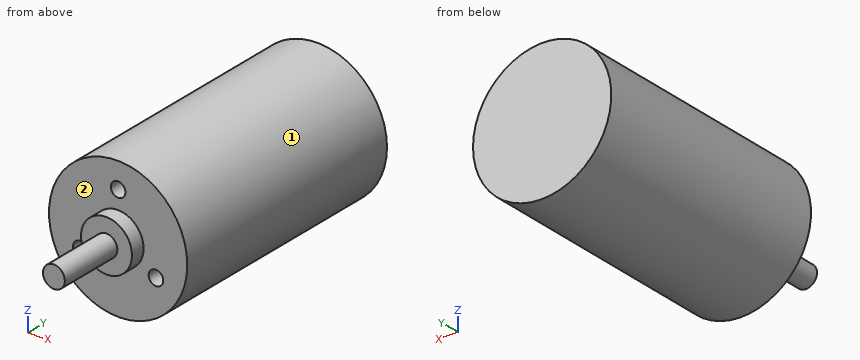
from build123d import *

# Parameters (mm, degrees)
F0_R     = 9.5
F1_DEPTH = 34.2
F2_R     = 3.5
F3_DEPTH = 2
F4_R     = 1.5
F5_DEPTH = 9
F7_D     = 2
F7_DEPTH = 3
F7_TIP   = 0.600860619


with BuildPart() as f1:
    # F0 (on Front) → F1 (new body)
    with BuildSketch(Plane.XZ):
        Circle(F0_R)
    extrude(amount=F1_DEPTH)

    # F2 (on face) → F3 (join)
    with BuildSketch(Plane.XZ.offset(34.2)):
        Circle(F2_R)
    extrude(amount=F3_DEPTH)

    # F4 (on face) → F5 (join)
    with BuildSketch(Plane.XZ.offset(36.2)):
        Circle(F4_R)
    extrude(amount=F5_DEPTH)

    # F7
    with Locations(Plane.XZ.offset(34.2)):
        with Locations((0, 6), (-5.1961524227, -3), (5.1961524227, -3)):
            Hole(F7_D / 2, depth=F7_DEPTH)
            with Locations((0, 0, -(F7_DEPTH + F7_TIP / 2))):  # 118° drill point
                Cone(0, F7_D / 2, F7_TIP, mode=Mode.SUBTRACT)


solid = f1.part
Could you check a few things on this model? Use its own coordinates, in mm. Face numbers are marked on the shaded views. A direction names the side the tool comes from. Coordinates: 2 decimals unless noted, no trailing zeros. Write each loop counter-clockwise with the first axis right and the second up, starting at its lowest first coordinate (ties: lowest second). Pieces come first, ordered by that corner, then holes. Notation, with made-up numbers: (82.25, -8.5) - (94.25, -8.5) arc R28 cw to (94.25, 16.5) - close; hole circle Ø9 at (32, 84). An arc over 180 degrees is marked (long way). Write item = value, one per line.
1) Will these pins go through, and if not, where does the flat tip stop? pin 1 Ø6 at (x, z) = (-1, 6.5) entering from -Y; pin 2 Ø6 at (y, z) = (-22, 7.5) entering from +X; pin 3 Ø1.5 at (x, y) = (4, -22) entering from +Z.
Result set:
pin_1 = -34.2
pin_2 = 8.37
pin_3 = 8.93
2) Please list where these lines run through material, in increasing order: line 1 (X direction, y = -33.15, z = -3); line 2 (Z direction, x = 0, y = -32.15); line 3 (Y direction, x = 0.75, z = -2.75). Write a range as [from, to].
Result set:
line_1 = [-9.01, -6.2], [-4.2, 4.2], [6.2, 9.01]
line_2 = [-9.5, 5], [7, 9.5]
line_3 = [-36.2, 0]
3) Suppose I cut it at B-B on y = -29.5. Please give me the cut outline in (x, z), plus the area to 3 significant figures.
Result set:
outline = circle Ø19 at (0, 0)
area = 284 mm2
4) Suppose I cut it at C-C on x = -2.5. Please give me the cut outline in (y, z).
Result set:
outline = (-36.2, -2.45) - (-34.2, -2.45) - (-34.2, -9.17) - (0, -9.17) - (0, 9.17) - (-34.2, 9.17) - (-34.2, 2.45) - (-36.2, 2.45) - close
5) Suppose I cut it at A-A on z = 0. Please give me the cut outline in (x, y).
Result set:
outline = (-9.5, -34.2) - (-3.5, -34.2) - (-3.5, -36.2) - (-1.5, -36.2) - (-1.5, -45.2) - (1.5, -45.2) - (1.5, -36.2) - (3.5, -36.2) - (3.5, -34.2) - (9.5, -34.2) - (9.5, 0) - (-9.5, 0) - close
6) For the marked faces 1 and 2, which set-ups out of +Z, -Z, +X, -X, +Y, -Y let a thin tool reach every point of the face, with its end or its side?
Result set:
face_1 = +Y, -Y
face_2 = -Y
7) Suppose I cut it at D-D on z = 3. Please give me the cut outline in (x, y).
Result set:
outline = (-9.01, -34.2) - (-1.8, -34.2) - (-1.8, -36.2) - (1.8, -36.2) - (1.8, -34.2) - (9.01, -34.2) - (9.01, 0) - (-9.01, 0) - close
